Autodesk Inventor part; units mm, degrees
ref_plane "YZ Plane" through (0, 0, 0) normal (1, 0, 0) x (0, 1, 0)
ref_plane "XZ Plane" through (0, 0, 0) normal (0, 1, 0) x (-1, 0, 0)
ref_plane "XY Plane" through (0, 0, 0) normal (0, 0, 1) x (1, 0, 0)
sketch "Sketch1" plane through (0, 0, 0) normal (0, 0, 1) x (1, 0, 0)
  line L0 (-45, 45) -> (-45, -45)
  line L1 (-45, -45) -> (-25, -45)
  line L2 (-25, -45) -> (45, 25)
  line L3 (45, 25) -> (45, 45)
  line L4 (45, 45) -> (-45, 45)
  point P0 (0, 0)
  point P1 (0, 45)
  point P2 (-45, 0)
  dimension "d0" = 20
  dimension "d1" = 20
  dimension "d2" = 90
  dimension "d3" = 90
extrude "Extrusion1" add sketch "Sketch1" along normal blind 5
sketch "Sketch2" plane through (0, 0, 5) normal (0, 0, 1) x (1, 0, 0)
  circle A0 centre (-11, 11) radius 2.5
  circle A1 centre (2, -2) radius 2.5
  line L0 (-25, -45) -> (45, 25)
  line L1 (45, 45) -> (-45, 45)
  line L2 (10, -10) -> (-45, 45) construction
  line L3 (-45, 45) -> (-45, -45)
  point P0 (0, 0)
  dimension "d6" = 5
  dimension "d7" = 34
  dimension "d8" = 13
extrude "Extrusion2" cut sketch "Sketch2" against normal blind 6
ref_plane "Work Plane2" through (-11, 11, 5) normal (0.7071, -0.7071, 0) x (0.7071, 0.7071, 0)
ref_plane "Work Plane1" through (-9.2322, 9.2322, 5) normal (0.7071, -0.7071, 0) x (0.7071, 0.7071, 0)
sketch "Sketch3" plane through (-11, 11, 5) normal (0.7071, -0.7071, 0) x (0.7071, 0.7071, 0)
  line L0 (-49.4975, 0) -> (49.4975, 0)
  line L1 (0, 11.5) -> (0, 0)
  line L2 (-9, 0) -> (0, 0)
  line L3 (-9, 0) -> (-4, 11.5)
  line L4 (-4, 11.5) -> (0, 11.5)
  point P0 (0, -5)
  dimension "d12" = 9
  dimension "d13" = 11.5
  dimension "d17" = 4
revolve "Revolution1" add sketch "Sketch3" angle 360 about axis through (-11, 11, 16.5) along (0, 0, -1)
sketch "Sketch4" plane through (-11, 11, 5) normal (0, 0, -1) x (-1, 0, 0)
  circle A0 centre (0, 0) radius 2.5
  point P0 (-11, -11)
extrude "Extrusion3" cut sketch "Sketch4" against normal up to next
sketch "Sketch5" plane through (0, 0, 5) normal (0, 0, 1) x (1, 0, 0)
  circle A0 centre (-35, -37) radius 2.1
  circle A1 centre (-35, -18) radius 2.1
  circle A2 centre (-35, 20) radius 2.1
  circle A3 centre (-20, 35) radius 2.1
  circle A4 centre (-1, 35) radius 2.1
  circle A5 centre (18, 35) radius 2.1
  circle A6 centre (37, 35) radius 2.1
  line L0 (-45, -45) -> (-25, -45)
  line L1 (45, 25) -> (45, 45)
  circle A7 centre (-35, 1) radius 2.1
  point P0 (0, 0)
  point P1 (45, 35)
  point P2 (-35, -45)
  point P3 (-35, -45)
  point P4 (-35, -45)
  dimension "d18" = 4.2
  dimension "d19" = 8
  dimension "d20" = 19
  dimension "d21" = 19
  dimension "d22" = 19
  dimension "d23" = 8
  dimension "d24" = 19
  dimension "d25" = 19
  dimension "d26" = 19
extrude "Extrusion4" cut sketch "Sketch5" against normal up to next
fillet "Fillet1" radius 2 1 edges at (-4.636, 17.364, 5)
sketch "Sketch7" plane through (0, 0, 0) normal (0, 0, -1) x (-1, 0, 0)
  line L0 (15.15, 13.396) -> (15.15, 8.604)
  line L1 (15.15, 8.604) -> (11, 6.208)
  line L2 (11, 6.208) -> (6.85, 8.604)
  line L3 (6.85, 8.604) -> (6.85, 13.396)
  line L4 (6.85, 13.396) -> (11, 15.792)
  line L5 (11, 15.792) -> (15.15, 13.396)
  circle A0 centre (11, 11) radius 2.5
  circle A1 centre (11, 11) radius 4.15 construction
  point P0 (0, 0)
  point P1 (15.15, 11)
  dimension "d30" = 8.3
  dimension "d32" = 8.3
extrude "Extrusion5" cut sketch "Sketch7" against normal blind 5
ref_plane "Work Plane4" through (2, -2, 5) normal (0.7071, -0.7071, 0) x (0.7071, 0.7071, 0)
ref_plane "Work Plane3" through (0.2322, -0.2322, 5) normal (0.7071, -0.7071, 0) x (0.7071, 0.7071, 0)
sketch "Sketch8" plane through (2, -2, 5) normal (0.7071, -0.7071, 0) x (0.7071, 0.7071, 0)
  line L0 (2.5, -5) -> (-2.5, -5)
  line L1 (-2.5, 0) -> (2.5, 0)
  line L2 (-2.5, 0) -> (2.5, 0)
  line L3 (-2.5, 0) -> (-7.5, 0)
  line L4 (-7.5, 0) -> (-4, 2)
  line L5 (-4, 2) -> (-2.5, 2)
  line L6 (-2.5, 0) -> (-2.5, 2)
  line L7 (0, 0) -> (0, 4.1579) construction
  point P0 (0, -5)
  dimension "d36" = 5
  dimension "d37" = 1.5
  dimension "d38" = 2
revolve "Revolution2" add sketch "Sketch8" angle 360 about axis through (2, -2, 5) along (0, 0, 1)
fillet "Fillet2" radius 5 5 edges at (-25, -45, 2.5) (-45, -45, 2.5) (45, 25, 2.5) (45, 45, 2.5) (-45, 45, 2.5)
sketch "Sketch9" plane through (0, 0, 5) normal (0, 0, 1) x (1, 0, 0)
  line L0 (-45, 40) -> (-45, -40)
  line L1 (-45, -13) -> (14.9089, -13)
  line L2 (14.9089, -13) -> (14.9089, -45)
  line L3 (14.9089, -45) -> (-45, -45)
  line L4 (-45, -45) -> (-45, -13)
  arc A0 (-27.0711, -45) -> (-23.5355, -43.5355) centre (-27.0711, -40) ccw
  point P0 (0, 0)
  point P1 (-25.1577, -44.6194)
  dimension "d44" = 32
extrude "Extrusion6" cut sketch "Sketch9" against normal up to next
equation "\"d21\" = d20"
equation "\"d22\" = d20"
equation "\"d24\" = d20"
equation "\"d25\" = d20"
equation "\"d26\" = d20"
properties part number "bracket-GT2-left"
The model under review builds one solid part; all positions refer to its coordinate system, in mm. A direction names the side the tool comes from. Round coordinates to 2 decimals unless told otherwise and drop trailing zeros. Loops run counter-clockwise (first coordinate to the right, second up) from the corner with the lowest first, then second, coordinate; pieces in that order, holes last. Notation, with made-up numbers: (35, 68) -> (43, 68) arc R19 ccw to (43, 74) -> close; hole circle Ø7 at (66, -10.5). An arc over 180 degrees is marked (long way). Answer as a JSON object with one key per item and string values. Group by question number.
1) For faces 1 (the face through (-1, 16, 0)), 2 (the face through (-9, 9, 5)), list the 3-axis set-ups (+Z, -Z, +X, -X, +Y, -Y) from which the entire face can be reached by the end or side of a thin tool; tool diameter is ignored.
2) We need section A-A on x = -35. Write out the cut boundary in (y, z), then the cut area to 3 significant figures.
3) We need section C-C on x = 18. Write out the cut boundary in (y, z).
4) Mouldability with a two-part tool opening along X and no side actions: class faces 3 (the face through (2, 1, 7)), 4 (the face through (-45, 14, 2)), 5 (the face through (-13.05, 14.61, 2.46)) as released by +X, released by -X, zero draft, split by the parting line, or undercut.
5) For line 1 (Y direction, x = -35, z = 1.7); line 2 (Y direction, x = -1, z = 1.2); line 3 (Z direction, x = 30.5, y = 40), list the stretches that pass through material, from the lowest coordinate up. Write a range as [from, to].
6) We need section D-D on z = 4. Give the number of separate pieces and of enclosed holes in the cut face, then the cut area to 3 significant figures.
7) We need section B-B on y = -2. Write out the cut boundary in (x, z).
8) For pin 1 Ø2 at (y, z) = (14.5, 5.5) entering from +X; pin 2 Ø6 at (x, y) = (-19, 28) entering from +Z; pin 3 Ø1 at (y, z) = (-2, 7) entering from +X (3 decimals), all flat-tipped, find the tip position at first contact; note any pin that passes through.
Result set:
{
 "1": {"face 1": "-Z, +X, -X, +Y, -Y", "face 2": "-Z"},
 "2": {"outline": "(-13, 0) -> (-1.1, 0) -> (-1.1, 5) -> (-13, 5) -> close; (3.1, 0) -> (17.9, 0) -> (17.9, 5) -> (3.1, 5) -> close; (22.1, 0) -> (45, 0) -> (45, 5) -> (22.1, 5) -> close", "area": "248 mm²"},
 "3": {"outline": "(-2, 0) -> (32.9, 0) -> (32.9, 5) -> (-2, 5) -> close; (37.1, 0) -> (45, 0) -> (45, 5) -> (37.1, 5) -> close"},
 "4": {"face 3": "zero draft", "face 4": "released by -X", "face 5": "undercut"},
 "5": {"line 1": "[-13, -1.1], [3.1, 17.9], [22.1, 45]", "line 2": "[-13, 32.9], [37.1, 45]", "line 3": "[0, 5]"},
 "6": {"separate pieces": "1", "enclosed holes": "8", "area": "4,320 mm²"},
 "7": {"outline": "(-45, 0) -> (-0.5, 0) -> (-0.5, 7) -> (-2, 7) -> (-5.5, 5) -> (-45, 5) -> close; (4.5, 0) -> (18, 0) -> (18, 5) -> (9.5, 5) -> (6, 7) -> (4.5, 7) -> close"},
 "8": {"pin 1": "x = 35.37", "pin 2": "z = 5", "pin 3": "x = 6.875"}
}
